Job drawing, mm, ordinate dimensions from the low corner. One solid piece. Coordinates: 2 decimals unless noted, no trailing zeros. Write each loop counter-clockwise with the first axis right and the second up, starting at its lowest first coordinate (ties: lowest second). Pieces come first, ordered by that corner, then holes. Notation, with made-up numbers: (12, -25.5) - (63, -25.5) arc R19 ccw to (63, -17.5) - close; hole circle Ø4 at (62, 41.5). An arc over 180 degrees is marked (long way). Put each result on its own line as item: value. Start each with the question number.
1. Saw through at B-B, the plane x = 217. Write the cut outline in (y, z).
2. Drill centre lines: L1, parallel to X at y = 44.6, z = 10; L2, parallel to Z at x = 310, y = 45.4; L3, parallel to Y at x = 100, z = 15.5. Where is each one in solid material? Low to high. Write a range as from..to.
3. Drop flat-ended pins along their axis: P1, Ø4, axis at x = 202.5, z = 17.5, coming from the -Y side; P2, Ø8, axis at x = 10, z = 10, coming from the +Y side; P3, Ø16, axis at x = 309.5, y = 29, coming from the -Z side; P4, Ø1, axis at y = 13, z = 17.5, coming from the -X side. Give the stop position or say it passes through.
4. Saw through at A-A, the plane y = 17.2. Write the cut outline in (x, z), plus the area to 4 significant figures.
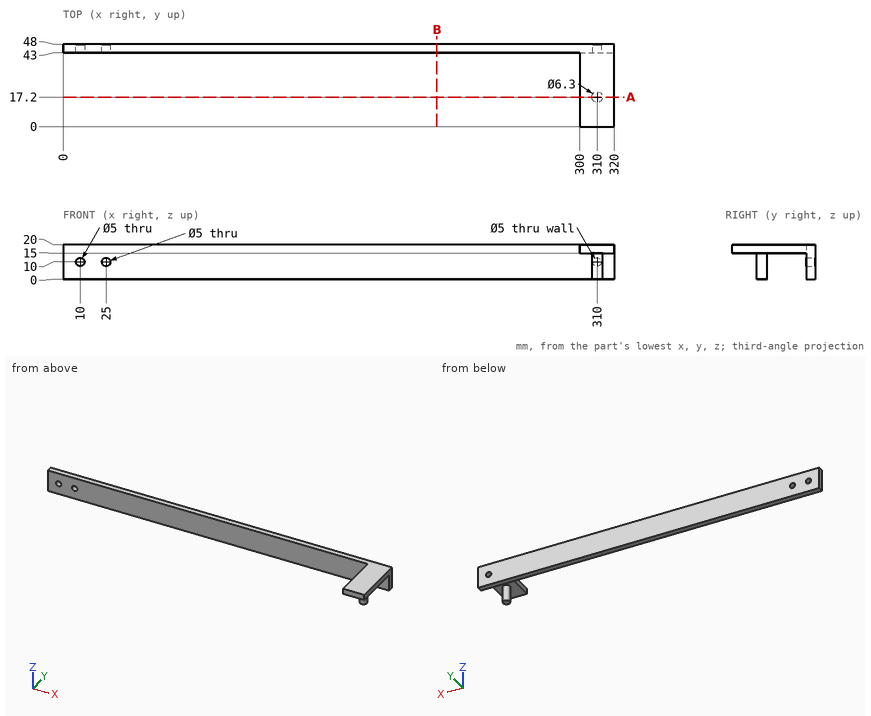
Final values:
1. outline: (43, 0) - (48, 0) - (48, 20) - (43, 20) - close
2. L1: x = 0..7.5, 12.5..22.5, 27.5..307.5, 312.5..320
2. L2: z = 0..7.5, 12.5..20
2. L3: y = 43..48
3. P1: stops at y = 43
3. P2: stops at y = 48
3. P3: stops at z = 15
3. P4: stops at x = 300
4. outline: (300, 15) - (306.85, 15) - (306.85, 0) - (313.15, 0) - (313.15, 15) - (320, 15) - (320, 20) - (300, 20) - close
4. area: 194.5 mm²
